```python
from build123d import *

# Parameters (mm, degrees)
F0_W     = 70
F0_H     = 30
F1_DEPTH = 41
F2_W     = 10
F2_H     = 10
F2_R     = 9.6999339811
F3_DEPTH = 41
F5_DEPTH = 70
F6_DEPTH = 70


with BuildPart() as f1:
    # F0 (on Front) → F1 (new body)
    with BuildSketch(Plane.XZ):
        with Locations((35, 15)):
            Rectangle(F0_W, F0_H)
    extrude(amount=-F1_DEPTH)

    # F2 (on face) → F3 (cut)
    with BuildSketch(Plane.XZ):
        with Locations((13, 15)):
            Rectangle(F2_W, F2_H)
        with Locations((35, 15)):
            Circle(F2_R)
        with Locations((57, 15)):
            Rectangle(F2_W, F2_H)
    extrude(amount=-F3_DEPTH, mode=Mode.SUBTRACT)

    # F4 (on face) → F5 (join)
    with BuildSketch(Plane.YZ.offset(70)):
        with BuildLine():
            ThreePointArc((54, 15), (50.1923881554, 24.1923881554), (41, 28))
            Line((41, 28), (41, 2))
            ThreePointArc((41, 2), (50.1923881554, 5.8076118446), (54, 15))
        make_face()
        with BuildLine():
            Line((41, 2), (41, 28))
            ThreePointArc((41, 28), (28, 15), (41, 2))
        make_face()
        with BuildLine():
            ThreePointArc((21, 0), (48.9056941504, -8.7170824513), (66, 15))
            ThreePointArc((66, 15), (48.9056941504, 38.7170824513), (21, 30))
            Line((21, 30), (41, 30))
            Line((41, 30), (41, 28))
            ThreePointArc((41, 28), (50.1923881554, 24.1923881554), (54, 15))
            ThreePointArc((54, 15), (50.1923881554, 5.8076118446), (41, 2))
            Line((41, 2), (41, 0))
            Line((41, 0), (21, 0))
        make_face()
    extrude(amount=-F5_DEPTH)

    # F4 (on face) → F6 (cut)
    with BuildSketch(Plane.YZ.offset(70)):
        with BuildLine():
            ThreePointArc((54, 15), (50.1923881554, 24.1923881554), (41, 28))
            Line((41, 28), (41, 2))
            ThreePointArc((41, 2), (50.1923881554, 5.8076118446), (54, 15))
        make_face()
        with BuildLine():
            Line((41, 2), (41, 28))
            ThreePointArc((41, 28), (28, 15), (41, 2))
        make_face()
    extrude(amount=-F6_DEPTH, mode=Mode.SUBTRACT)


solid = f1.part
```
Could you check a few things on this model? Use its own coordinates, in mm. A direction names the side the tool comes from. Coordinates: 2 decimals unless noted, no trailing zeros. Order: outer loops, then holes, each group sorted by start corner. A loop starts at its lowest first (then second) coordinate and runs counter-clockwise, first axis right, second up. Notation, with made-up numbers: M -37,-3.75 L 16,-3.75 A15 cw 16,6.25 Z; hole C 34.25,38.5 d7. An arc over 180 degrees is marked long. Use one line per item in the form item = value. Start each with the question number.
1. Suppose I cut it at B-B on z = 13.5. Write out the boundary of the cut face in (x, y).
2. On a 3-axis mill with a long thin cutter (end or side, diameter ignored), from which of +Z, -Z, +X, -X, +Y, -Y can I reach the whole of each face in a straight line? I mean faces 1 (the flat face through (13, 14, 20)), 2 (the flat face through (35, 10, 30)), 3 (the flat face through (35, 0, 5)). Say none if no direction works.
3. Suppose I cut it at C-C on x = 35. Write out the boundary of the cut face in (y, z), then the cut area to 3 significant figures.
4. We'd pull the mould along X, two halves only. Please class faces 4 (the flat face through (35, 10, 0)), 5 (the flat face through (13, 14, 10)), 6 (the flat face through (70, 25, 15)): +X half, -X half, draft (parallel to the pull), parting line (faces both ways), or undercut.
5. Suppose I cut it at D-D on y = 53. Write out the boundary of the cut face in (x, z).
6. For pin 1 (12 mm diameter, centred on y = 32, z = 12.5, fed in from -X); pin 2 (8 mm diameter, centred on x = 10.5, z = 6.5, fed in from +Y); pin 3 (1 mm diameter, centred on x = 62.5, y = 10, fed in from +Z); pin 4 (6 mm diameter, centred on y = 37.5, z = 8.5, fed in from -X), each with a flat end and sliding along its axis, tell me the tip position at first contact or that it passes through.
7. Suppose I cut it at A-A on y = 11.5. Write out the boundary of the cut face in (x, z), then the cut area to 3 significant figures.
8. Please list where these lines run through material, in increasing order: line 1 (X direction, y = 7, z = 15); line 2 (Z direction, x = 35, y = 21); line 3 (Z direction, x = 10, y = 11).
Geometry says:
q1.outline = M 0,0 L 8,0 L 8,28.09 L 0,28.09 Z; M 0,53.91 L 70,53.91 L 70,65.95 L 0,65.95 Z; M 18,0 L 25.42,0 L 25.42,28.09 L 18,28.09 Z; M 44.58,0 L 52,0 L 52,28.09 L 44.58,28.09 Z; M 62,0 L 70,0 L 70,28.09 L 62,28.09 Z
q2.face_1 = -Y
q2.face_2 = +Z, +X, -X, -Y
q2.face_3 = +Z, -Z, +X, -X, -Y
q3.outline = M 0,0 L 21,0 A25 ccw long 21,30 L 0,30 L 0,24.7 L 32.34,24.7 A13 cw long 32.34,5.3 L 0,5.3 Z
q3.area = 1,390 mm^2
q4.face_4 = draft
q4.face_5 = undercut
q4.face_6 = +X half
q5.outline = M 0,-6.93 L 70,-6.93 L 70,10 L 0,10 Z; M 0,20 L 70,20 L 70,36.93 L 0,36.93 Z
q6.pin_1 = 0
q6.pin_2 = 65.59
q6.pin_3 = 30
q6.pin_4 = through
q7.outline = M 0,0 L 70,0 L 70,30 L 0,30 Z; hole M 8,10 L 18,10 L 18,20 L 8,20 Z; hole C 35,15 d19.4; hole M 52,10 L 62,10 L 62,20 L 52,20 Z
q7.area = 1,600 mm^2
q8.line_1 = 0 to 8, 18 to 25.3, 44.7 to 52, 62 to 70
q8.line_2 = 0 to 5.3, 24.7 to 30
q8.line_3 = 0 to 10, 20 to 30
